Here's the drawing with two shaded views (mm, measured from the low corner). I have some questions. Round coordinates to 2 decimals unless told otherwise and drop trailing zeros. Order: outer loops, then holes, each group sorted by start corner. A loop starts at its lowest first (then second) coordinate and runs counter-clockwise, first axis right, second up. Notation, with made-up numbers: (-0.75, 3.25) - (8.25, 3.25) arc R24 ccw to (8.25, 27.25) - close; hole circle Ø5 at (69, 80). An arc over 180 degrees is marked (long way). Return JSON: item names as keys, results as strings. Group by question number.
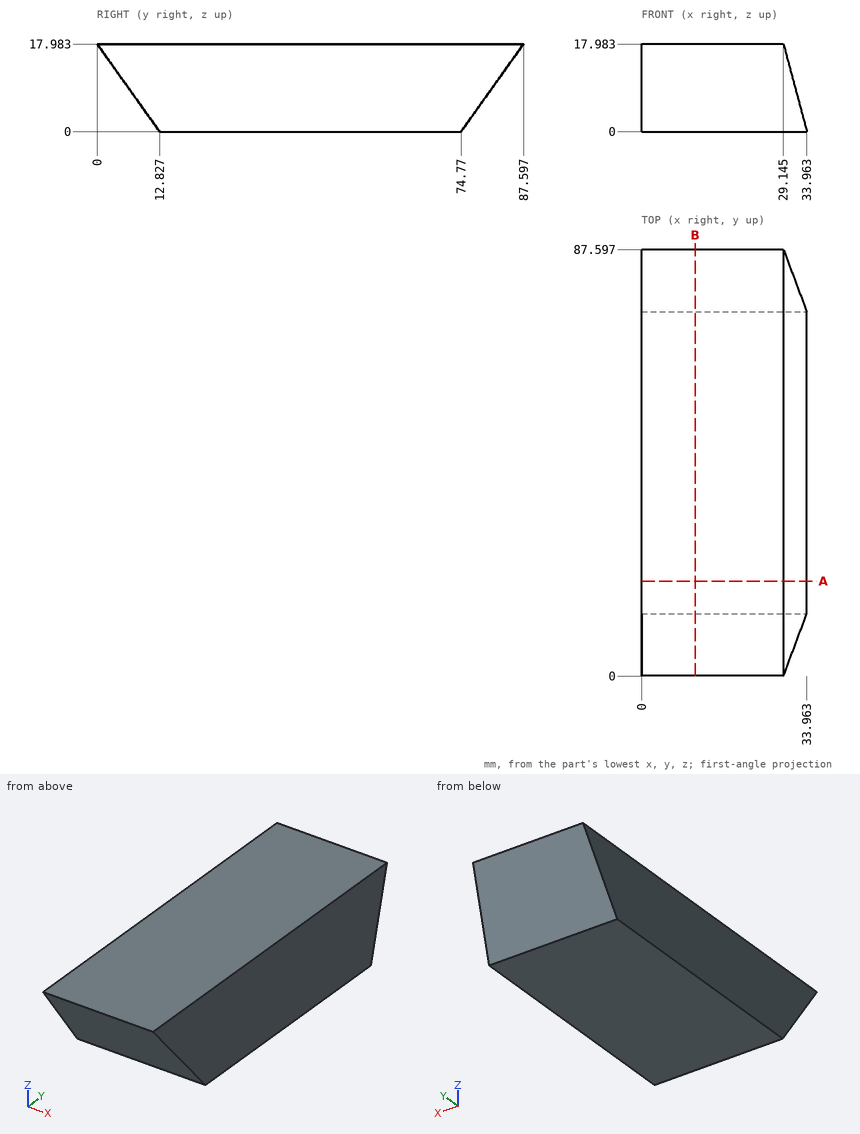
1) If I drill on line 1 along Y through (x, z) = (31.5, 5.75) (1 decimal); line 2 along Y through (x, z) = (11, 17.25) (1 decimal); line 3 along X through (y, z) = (68.5, 2.25), over which ranges is the centre line in solid material (lowest first)? Write a range as from..to.
2) I want a section at A-A, the plane y = 19.5. List the corners of the cut face in (x, z) for me (1 decimal).
3) Will these pins go through, and if not, where does the flat tip stop? pin 1 (1 mm diameter, centred on y = 56.5, z = 13, fed in from +X); pin 2 (2 mm diameter, centred on x = 12, z = 5.5, fed in from +Y); pin 3 (2 mm diameter, centred on x = 19.5, z = 13.5, fed in from +Y).
4) I want a section at B-B, the plane x = 11. List the corners of the cut face in (y, z) for me, plus the area to 3 significant figures.
Outcome:
{
 "1": {"line 1": "8.7..78.9", "line 2": "0.5..87.1", "line 3": "0..33.36"},
 "2": {"outline": "(0, 0) - (34, 0) - (29.1, 18) - (0, 18) - close"},
 "3": {"pin 1": "x = 30.61", "pin 2": "y = 79.41", "pin 3": "y = 85.11"},
 "4": {"outline": "(0, 17.98) - (12.83, 0) - (74.77, 0) - (87.6, 17.98) - close", "area": "1,340 mm^2"}
}
